Source: CAD feature listing. Evaluate the final solid. Frame: model axes, mm. Coordinates: 2 decimals unless noted, no trailing zeros. Write each loop counter-clockwise with the first axis right and the second up, starting at its lowest first coordinate (ties: lowest second). Pieces come first, ordered by that corner, then holes. Notation, with made-up numbers: M -37.5,72.25 L -13.5,72.25 A13 cw -13.5,97.25 Z; hole C -10.75,20 d3. An arc over 180 degrees is marked long. Answer as CSV lines item,"result". Start each with the question number.
1. Mould query, pull axis X, two halves, no side actions, for faces 1 (the face through (15.3, 6.4, 33.1)), 2 (the face through (-342.9, 6, 2)), 3 (the face through (-5, 6, -152.4)). Classes: pulls with the +X half, pulls with the -X half, needs draft (parallel to the pull), parting line crosses it, or undercut.
2. Section A-A on x = -165.1. Return the cut outline in (y, z), plus the area to 3 significant figures.
3. Section B-B on y = 9.75. Count the separate pieces of the cut face and the enclosed holes in it, plus the area to 3 significant figures.
4. Line query: probe 1 along Z at (x, y) = (-292.1, 9.75); probe 2 along Z at (x, y) = (37, 6). Output: solid intervals per line, ascending. Write a range as [from, to].
```python
from build123d import *

# Parameters (mm, degrees)
SKETCH1_W           = 685.8
SKETCH1_H           = 304.8
BOSS_EXTRUDE1_DEPTH = 12.7
SKETCH2_R           = 12.7
CUT_EXTRUDE1_DEPTH  = 13.7


with BuildPart() as part:
    # Sketch1 → Boss-Extrude1 (new body)
    with BuildSketch(Plane(origin=(0, 0, 0), x_dir=(1, 0, 0), z_dir=(0, 1, 0))):
        Rectangle(SKETCH1_W, SKETCH1_H)
    extrude(amount=BOSS_EXTRUDE1_DEPTH)

    # Sketch2 → Cut-Extrude1 (cut, through all)
    with BuildSketch(Plane(origin=(0, 12.7, 0), x_dir=(1, 0, 0), z_dir=(0, 1, 0))):
        with Locations((-292.1, 101.6)):
            Circle(SKETCH2_R)
        with Locations((-228.6, 101.6)):
            Circle(SKETCH2_R)
        with Locations((-165.1, 101.6)):
            Circle(SKETCH2_R)
        with Locations((-101.6, 101.6)):
            Circle(SKETCH2_R)
        with Locations((-38.1, 101.6)):
            Circle(SKETCH2_R)
        with Locations((25.4, 101.6)):
            Circle(SKETCH2_R)
        with Locations((88.9, 101.6)):
            Circle(SKETCH2_R)
        with Locations((152.4, 101.6)):
            Circle(SKETCH2_R)
        with Locations((215.9, 101.6)):
            Circle(SKETCH2_R)
        with Locations((279.4, 101.6)):
            Circle(SKETCH2_R)
        with Locations((-228.6, 38.1)):
            Circle(SKETCH2_R)
        with Locations((-165.1, 38.1)):
            Circle(SKETCH2_R)
        with Locations((-101.6, 38.1)):
            Circle(SKETCH2_R)
        with Locations((-38.1, 38.1)):
            Circle(SKETCH2_R)
        with Locations((25.4, 38.1)):
            Circle(SKETCH2_R)
        with Locations((88.9, 38.1)):
            Circle(SKETCH2_R)
        with Locations((152.4, 38.1)):
            Circle(SKETCH2_R)
        with Locations((215.9, 38.1)):
            Circle(SKETCH2_R)
        with Locations((279.4, 38.1)):
            Circle(SKETCH2_R)
        with Locations((-228.6, -25.4)):
            Circle(SKETCH2_R)
        with Locations((-165.1, -25.4)):
            Circle(SKETCH2_R)
        with Locations((-101.6, -25.4)):
            Circle(SKETCH2_R)
        with Locations((-38.1, -25.4)):
            Circle(SKETCH2_R)
        with Locations((25.4, -25.4)):
            Circle(SKETCH2_R)
        with Locations((88.9, -25.4)):
            Circle(SKETCH2_R)
        with Locations((152.4, -25.4)):
            Circle(SKETCH2_R)
        with Locations((215.9, -25.4)):
            Circle(SKETCH2_R)
        with Locations((279.4, -25.4)):
            Circle(SKETCH2_R)
        with Locations((-228.6, -88.9)):
            Circle(SKETCH2_R)
        with Locations((-165.1, -88.9)):
            Circle(SKETCH2_R)
        with Locations((-101.6, -88.9)):
            Circle(SKETCH2_R)
        with Locations((-38.1, -88.9)):
            Circle(SKETCH2_R)
        with Locations((25.4, -88.9)):
            Circle(SKETCH2_R)
        with Locations((88.9, -88.9)):
            Circle(SKETCH2_R)
        with Locations((152.4, -88.9)):
            Circle(SKETCH2_R)
        with Locations((215.9, -88.9)):
            Circle(SKETCH2_R)
        with Locations((279.4, -88.9)):
            Circle(SKETCH2_R)
        with Locations((-292.1, 38.1)):
            Circle(SKETCH2_R)
        with Locations((-292.1, -25.4)):
            Circle(SKETCH2_R)
        with Locations((-292.1, -88.9)):
            Circle(SKETCH2_R)
    extrude(amount=-CUT_EXTRUDE1_DEPTH, mode=Mode.SUBTRACT)


solid = part.part
```
Values:
1,face 1,"undercut"
1,face 2,"pulls with the -X half"
1,face 3,"needs draft"
2,outline,"M 0,-152.4 L 12.7,-152.4 L 12.7,-114.3 L 0,-114.3 Z; M 0,-88.9 L 12.7,-88.9 L 12.7,-50.8 L 0,-50.8 Z; M 0,-25.4 L 12.7,-25.4 L 12.7,12.7 L 0,12.7 Z; M 0,38.1 L 12.7,38.1 L 12.7,76.2 L 0,76.2 Z; M 0,101.6 L 12.7,101.6 L 12.7,152.4 L 0,152.4 Z"
2,area,"2,580 mm²"
3,separate pieces,"1"
3,enclosed holes,"40"
3,area,"189,000 mm²"
4,probe 1,"[-152.4, -114.3], [-88.9, -50.8], [-25.4, 12.7], [38.1, 76.2], [101.6, 152.4]"
4,probe 2,"[-152.4, -106.77], [-96.43, -43.27], [-32.93, 20.23], [30.57, 83.73], [94.07, 152.4]"
